Autodesk Inventor part; units mm, degrees
ref_plane "YZ Plane" through (0, 0, 0) normal (1, 0, 0) x (0, 1, 0)
ref_plane "XZ Plane" through (0, 0, 0) normal (0, 1, 0) x (-1, 0, 0)
ref_plane "XY Plane" through (0, 0, 0) normal (0, 0, 1) x (1, 0, 0)
sketch "Sketch1" plane through (0, 0, 0) normal (0, 0, 1) x (1, 0, 0)
  circle A0 centre (0, 0) radius 3.6
  dimension "d0" = 7.2
extrude "Extrusion1" add sketch "Sketch1" along normal blind 53.4
sketch "Sketch2" plane through (0, 0, 53.4) normal (0, 0, 1) x (1, 0, 0)
  circle A0 centre (0, 0) radius 1.5
  circle A1 centre (0, 0) radius 3.6
  dimension "d3" = 3
  dimension "d4" = 7.2
extrude "Extrusion2" cut sketch "Sketch2" against normal blind 22
sketch "Sketch3" plane through (0, 0, 31.4) normal (0, 0, 1) x (1, 0, 0)
  circle A0 centre (0, 0) radius 3.6
  circle A1 centre (0, 0) radius 2.35
  dimension "d7" = 7.2
  dimension "d8" = 4.7
chamfer "Chamfer1" distance 4.5 distance2 1.25 1 edges at (-3.6, 0, 31.4) measured on face at (3.5534, -0.5775, 20.9333)
properties part number "Solenoid_pin"
Geometry check sheet. Reference: the model listing, model coordinates, mm. A direction names the side the tool comes from. Give positions to 0.01 mm unless a question says otherwise; leave off trailing zeros. Order: outer loops, then holes, each group sorted by start corner. A loop starts at its lowest first (then second) coordinate and runs counter-clockwise, first axis right, second up.
1. Access from +Z, -Z, +X, -X, +Y, -Y to the whole of each face (thin tool, end or side, straight path). Record for faces 1 (the face through (-1.5, 0.07, 42.55)), 2 (the face through (0, 0, 0)).
Completed:
face 1: +Z
face 2: -Z, +X, -X, +Y, -Y
2. Scan lines: line 1 (Z direction, x = 0.5, y = 2); line 2 (X direction, y = 1.25, z = 45); line 3 (Y direction, x = -2.5, z = 20.5). Record each from-to range of solid material in increasing order.
Completed:
line 1: z = 0 to 31.4
line 2: x = -0.83 to 0.83
line 3: y = -2.59 to 2.59
3. Sectioned sample at A-A (y = 0). Record the boundary of the cut face in (x, z), then the cut area to 3 significant figures.
Completed:
outline: (-3.6, 0) - (3.6, 0) - (3.6, 26.9) - (2.35, 31.4) - (1.5, 31.4) - (1.5, 53.4) - (-1.5, 53.4) - (-1.5, 31.4) - (-2.35, 31.4) - (-3.6, 26.9) - close
area: 286 mm2
4. Depth check by flat-ended pin: pin 1 (2 mm diameter, centred on x = -2, z = 21, fed in from +Y); pin 2 (4 mm diameter, centred on x = -1.5, y = -1.5, fed in from -Z); pin 3 (1.5 mm diameter, centred on y = -0.5, z = 28, fed in from -X); pin 4 (1.5 mm diameter, centred on x = -1, z = 10, fed in from -Y). Enter the tip coordinate at first touch or a pass-through.
Completed:
pin 1: stops at y = 3.46
pin 2: stops at z = 0
pin 3: stops at x = -3.48
pin 4: stops at y = -3.59
5. Sectioned sample at C-C (z = 33). Record the boundary of the cut face in (x, y).
Completed:
outline: circle Ø3 at (0, 0)
6. Sectioned sample at D-D (z = 9). Record the boundary of the cut face in (x, y), then the cut area to 3 significant figures.
Completed:
outline: circle Ø7.2 at (0, 0)
area: 40.7 mm2
